from build123d import *

# Parameters (mm, degrees)
CYLINDER131_R               = 1.5
CYLINDER131_DEPTH           = 4
CYLINDER129_R               = 1.5
CYLINDER129_DEPTH           = 100
BOX043_W                    = 2
BOX043_H                    = 6
BOX043_DEPTH                = 6
COMPOUND160_PLACEMENT_ANGLE = 90
CYLINDER127_R               = 1.5
CYLINDER127_DEPTH           = 4
CYLINDER130_R               = 1.5
CYLINDER130_DEPTH           = 100
BOX042_W                    = 2
BOX042_H                    = 6
BOX042_DEPTH                = 6
COMPOUND161_PLACEMENT_ANGLE = 90
CYLINDER128_R               = 52
CYLINDER128_DEPTH           = 20
BOX044_W                    = 108
BOX044_H                    = 36
BOX044_DEPTH                = 20


with BuildPart() as obj1:
    # Cylinder131 → Cylinder131 (new body)
    with BuildSketch(Plane(origin=(-4, 3, 3), x_dir=(0, 0, -1), z_dir=(1, 0, 0))):
        Circle(CYLINDER131_R)
    extrude(amount=CYLINDER131_DEPTH)


with BuildPart() as obj2:
    # Cylinder129 → Cylinder129 (new body)
    with BuildSketch(Plane(origin=(2, 3, 3), x_dir=(0, 0, -1), z_dir=(1, 0, 0))):
        Circle(CYLINDER129_R)
    extrude(amount=CYLINDER129_DEPTH)


with BuildPart() as compound160:
    # Box043 → Box043 (new body)
    with BuildSketch(Plane.XY):
        with Locations((1, 3)):
            Rectangle(BOX043_W, BOX043_H)
    extrude(amount=BOX043_DEPTH)

    # Compound160: union obj1, obj2
    add(obj1.part)
    add(obj2.part)


with BuildPart() as compound160_1:
    # Compound160 placement: moved
    add(compound160.part.moved(Location((-54, 166, 27))).rotate(Axis((-54, 166, 27), (0, 0, -1)), COMPOUND160_PLACEMENT_ANGLE))


with BuildPart() as obj3:
    # Cylinder127 → Cylinder127 (new body)
    with BuildSketch(Plane(origin=(-4, 3, 3), x_dir=(0, 0, -1), z_dir=(1, 0, 0))):
        Circle(CYLINDER127_R)
    extrude(amount=CYLINDER127_DEPTH)


with BuildPart() as obj4:
    # Cylinder130 → Cylinder130 (new body)
    with BuildSketch(Plane(origin=(2, 3, 3), x_dir=(0, 0, -1), z_dir=(1, 0, 0))):
        Circle(CYLINDER130_R)
    extrude(amount=CYLINDER130_DEPTH)


with BuildPart() as fusion005:
    # Box042 → Box042 (new body)
    with BuildSketch(Plane.XY):
        with Locations((1, 3)):
            Rectangle(BOX042_W, BOX042_H)
    extrude(amount=BOX042_DEPTH)

    # Compound161: union obj3, obj4
    add(obj3.part)
    add(obj4.part)


with BuildPart() as fusion005_1:
    # Compound161 placement: moved
    add(fusion005.part.moved(Location((48, 166, 27))).rotate(Axis((48, 166, 27), (0, 0, -1)), COMPOUND161_PLACEMENT_ANGLE))

    # Fusion005: union Compound160
    add(compound160_1.part)


with BuildPart() as obj5:
    # Cylinder128 → Cylinder128 (new body)
    with BuildSketch(Plane.XY.offset(20)):
        Circle(CYLINDER128_R)
    extrude(amount=CYLINDER128_DEPTH)


with BuildPart() as cut060:
    # Box044 → Box044 (new body)
    with BuildSketch(Plane(origin=(-54, -53, 20), x_dir=(1, 0, 0), z_dir=(0, 0, 1))):
        with Locations((54, 18)):
            Rectangle(BOX044_W, BOX044_H)
    extrude(amount=BOX044_DEPTH)

    # Cut061: cut obj5
    add(obj5.part, mode=Mode.SUBTRACT)

    # Cut060: cut Fusion005
    add(fusion005_1.part, mode=Mode.SUBTRACT)


with BuildPart() as cut060_1:
    # Cut060 placement: moved
    add(cut060.part.moved(Location((0, 0, -20))))


solid = cut060_1.part
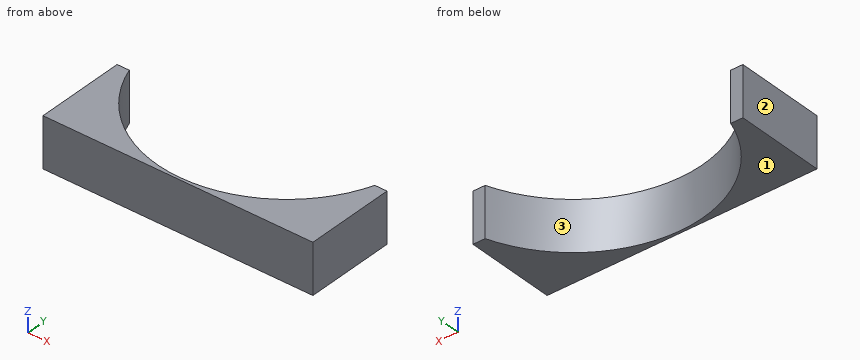
CAD build for the part. Positions are in the model's coordinates, mm. Face numbers are marked on the shaded views. Give positions to 0.01 mm unless a question says otherwise; leave off trailing zeros. Write each loop counter-clockwise with the first axis right and the second up, starting at its lowest first coordinate (ties: lowest second). Pieces come first, ordered by that corner, then holes. Notation, with made-up numbers: (57, -24.75) - (98, -24.75) arc R28 ccw to (98, -0.75) - close; hole circle Ø5 at (64, -3). An arc over 180 degrees is marked (long way). Answer as CSV lines item,"result".
Q1. Band-saw the part on C-C (y = -37). Give the cut face in (x, z).
Result set:
outline,"(-54, 0) - (-36.54, 0) - (-36.54, 20) - (-54, 20) - close; (36.54, 0) - (54, 0) - (54, 20) - (36.54, 20) - close"
Q2. Drill centre lines: line 1 (X direction, y = -44, z = 13.5); line 2 (X direction, y = -27, z = 15.5); line 3 (Y direction, x = 17, z = 5.5). Where is each one in solid material? Low to high. Write a range as from..to.
Result set:
line 1,"-54..-27.71, 27.71..54"
line 2,"-54..-44.44, 44.44..54"
line 3,"-53..-49.14"
Q3. Flat gauge pins, fed straight in: pin 1 Ø12 at (x, y) = (13, -42) entering from +Z; pin 2 Ø12 at (x, z) = (24, 7.5) entering from +Y. Where does each tip first touch, or does it go through?
Result set:
pin 1,"through"
pin 2,"y = -42.47"
Q4. Band-saw the part on B-B (z = 5.25). Give the cut face in (x, y).
Result set:
outline,"(-54, -53) - (54, -53) - (54, -17) - (49.14, -17) arc R52 cw to (-49.14, -17) - (-54, -17) - close"
Q5. Pull direction X, two halves, no side cores. Call the marked faces 1, 2 and 3: released by +X, released by -X, zero draft, split by the parting line, or undercut.
Result set:
face 1,"zero draft"
face 2,"released by -X"
face 3,"undercut"
Q6. Band-saw the part on A-A (y = -48). Give the cut face in (x, z), and give its area (3 significant figures).
Result set:
outline,"(-54, 0) - (-20, 0) - (-20, 20) - (-54, 20) - close; (20, 0) - (54, 0) - (54, 20) - (20, 20) - close"
area,"1,360 mm²"
Q7. Band-saw the part on D-D (x = -23.5). Give the cut face in (y, z), and give its area (3 significant figures).
Result set:
outline,"(-53, 0) - (-46.39, 0) - (-46.39, 20) - (-53, 20) - close"
area,"132 mm²"
